Source: CAD feature listing. Evaluate the final solid. Frame: model axes, mm. Face numbers are marked on the shaded views. A direction names the side the tool comes from. Give positions to 0.01 mm unless a question says otherwise; leave off trailing zeros. Order: outer loops, then holes, each group sorted by start corner. A loop starts at its lowest first (then second) coordinate and runs counter-clockwise, first axis right, second up. Notation, with made-up numbers: (77, 19.25) - (116, 19.25) arc R23 cw to (116, 29.25) - close; hole circle Ø8 at (44.5, 71.5). An arc over 180 degrees is marked (long way). Answer as CSV lines item,"result".
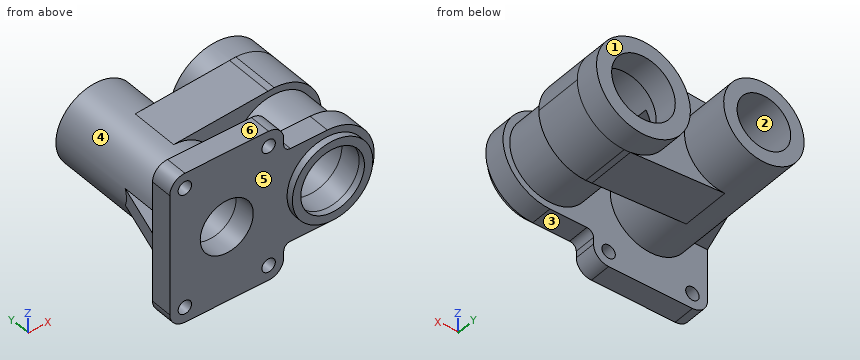
```python
from build123d import *

# Parameters (mm, degrees)
SKETCH3_W                 = 68
SKETCH3_H                 = 90
BOSS_EXTRUDE1_DEPTH       = 13
FILLET2_R                 = 4
FILLET3_R                 = 9
SKETCH5_R                 = 4
CUT_EXTRUDE1_DEPTH        = 100.689518005
SKETCH6_R                 = 24
SKETCH6_R_2               = 16
BOSS_EXTRUDE2_DEPTH       = 41.064418341
SKETCH7_R                 = 24
SKETCH7_R_2               = 19
BOSS_EXTRUDE3_DEPTH       = 17
BOSS_EXTRUDE4_START       = 28
SKETCH7_2_R               = 24
SKETCH7_2_R_2             = 19
BOSS_EXTRUDE4_DEPTH       = 28
BOSS_EXTRUDE11_DEPTH      = 28
BOSS_EXTRUDE11_DEPTH_BACK = 1
SKETCH8_R                 = 24
SKETCH8_R_2               = 16
SKETCH9_W                 = 95
SKETCH9_H                 = 12
CUT_EXTRUDE2_DEPTH        = 12.5
SKETCH10_R                = 24
SKETCH10_R_2              = 16
BOSS_EXTRUDE12_DEPTH      = 29.5
SKETCH12_R                = 28
SKETCH12_R_2              = 19
BOSS_EXTRUDE13_DEPTH      = 14.5
RIB1_REACH                = 141.539
SKETCH13_WALL_W           = 318.21240823
SKETCH13_WALL_H           = 10
SKETCH15_R                = 15.829166104
SKETCH15_R_2              = 19
CUT_EXTRUDE5_DEPTH        = 140.539420953


with BuildPart() as part:
    # Sketch3 → Boss-Extrude1 (new body)
    with BuildSketch(Plane(origin=(0, 0, 0), x_dir=(1, 0, 0), z_dir=(0, 1, 0))):
        Rectangle(SKETCH3_W, SKETCH3_H)
        with BuildLine():
            Line((60, 28), (34, 28))
            Line((34, 28), (34, -28))
            Line((34, -28), (60, -28))
            ThreePointArc((60, -28), (88, 0), (60, 28))
        make_face()
    extrude(amount=BOSS_EXTRUDE1_DEPTH)

    # Fillet2
    fillet2_edges = [part.edges().sort_by_distance(p)[0] for p in [
        (34, 6.5, -28),
        (34, 6.5, 28),
    ]]
    fillet(fillet2_edges, radius=FILLET2_R)

    # Fillet3
    fillet3_edges = [part.edges().sort_by_distance(p)[0] for p in [
        (34, 6.5, 45),
        (-34, 6.5, 45),
        (-34, 6.5, -45),
        (34, 6.5, -45),
    ]]
    fillet(fillet3_edges, radius=FILLET3_R)

    # Sketch5 → Cut-Extrude1 (cut, through all)
    with BuildSketch(Plane(origin=(0, 13, 0), x_dir=(1, 0, 0), z_dir=(0, 1, 0))):
        with Locations(Location((-25, 36, 0), (0, 0, 270))):
            Circle(SKETCH5_R)
        with Locations(Location((25, 36, 0), (0, 0, 270))):
            Circle(SKETCH5_R)
        with Locations(Location((-25, -36, 0), (0, 0, 270))):
            Circle(SKETCH5_R)
        with Locations(Location((25, -36, 0), (0, 0, 270))):
            Circle(SKETCH5_R)
    extrude(amount=-CUT_EXTRUDE1_DEPTH, mode=Mode.SUBTRACT)

    # Sketch6 → Boss-Extrude2 (add)
    with BuildSketch(Plane(origin=(0, 0, 0), x_dir=(1, 0, 0), z_dir=(0, 1, 0))):
        with Locations(Location((0, 0, 0), (0, 0, 270))):
            Circle(SKETCH6_R)
        with Locations(Location((0, 0, 0), (0, 0, 270))):
            Circle(SKETCH6_R_2, mode=Mode.SUBTRACT)
    extrude(amount=BOSS_EXTRUDE2_DEPTH)

    # Sketch7 → Boss-Extrude3 (add)
    with BuildSketch(Plane(origin=(0, 13, 0), x_dir=(1, 0, 0), z_dir=(0, 1, 0))):
        with Locations(Location((60, 0, 0), (0, 0, 270))):
            Circle(SKETCH7_R)
        with Locations(Location((60, 0, 0), (0, 0, 270))):
            Circle(SKETCH7_R_2, mode=Mode.SUBTRACT)
    extrude(amount=-BOSS_EXTRUDE3_DEPTH)

    # Sketch7_2 → Boss-Extrude4 (add)
    with BuildSketch(Plane(origin=(0, 13, 0), x_dir=(1, 0, 0), z_dir=(0, 1, 0)).offset(BOSS_EXTRUDE4_START)):
        with Locations(Location((60, 0, 0), (0, 0, 270))):
            Circle(SKETCH7_2_R)
        with Locations(Location((60, 0, 0), (0, 0, 270))):
            Circle(SKETCH7_2_R_2, mode=Mode.SUBTRACT)
    extrude(amount=-BOSS_EXTRUDE4_DEPTH)

    # Sketch8 → Boss-Extrude11 (add, two sides: drawn at the far end of the back side and taken through both)
    # profile 1 of 3: a face of its own
    with BuildSketch(Plane(origin=(0, 41, 0), x_dir=(1, 0, 0), z_dir=(0, 1, 0)).offset(-BOSS_EXTRUDE11_DEPTH_BACK)):
        with Locations(Location((0, 0, 0), (0, 0, 270))):
            Circle(SKETCH8_R)
        with Locations(Location((0, 0, 0), (0, 0, 270))):
            Circle(SKETCH8_R_2, mode=Mode.SUBTRACT)
    # profile 2 of 3: a face of its own
    with BuildSketch(Plane(origin=(0, 41, 0), x_dir=(1, 0, 0), z_dir=(0, 1, 0)).offset(-BOSS_EXTRUDE11_DEPTH_BACK)):
        with BuildLine():
            Line((60, 28), (56.283185841, 27.752212389))
            ThreePointArc((56.283185841, 27.752212389), (32, 0), (56.283185841, -27.752212389))
            Line((56.283185841, -27.752212389), (60, -28))
            ThreePointArc((60, -28), (79.798989873, -19.798989873), (88, 0))
            ThreePointArc((88, 0), (79.798989873, 19.798989873), (60, 28))
        make_face()
        with Locations(Location((60, 0, 0), (0, 0, 270))):
            Circle(SKETCH8_R, mode=Mode.SUBTRACT)
    # profile 3 of 3: a face of its own
    with BuildSketch(Plane(origin=(0, 41, 0), x_dir=(1, 0, 0), z_dir=(0, 1, 0)).offset(-BOSS_EXTRUDE11_DEPTH_BACK)):
        with BuildLine():
            Line((56.283185841, 27.752212389), (0, 24))
            ThreePointArc((0, 24), (16.970562748, 16.970562748), (24, 0))
            ThreePointArc((24, 0), (16.970562748, -16.970562748), (0, -24))
            Line((0, -24), (56.283185841, -27.752212389))
            ThreePointArc((56.283185841, -27.752212389), (32, 0), (56.283185841, 27.752212389))
        make_face()
    extrude(amount=BOSS_EXTRUDE11_DEPTH + BOSS_EXTRUDE11_DEPTH_BACK)

    # Sketch9 → Cut-Extrude2 (cut, symmetric)
    with BuildSketch(Plane.XY):
        with Locations((31.5, 53.5)):
            Rectangle(SKETCH9_W, SKETCH9_H)
    extrude(amount=CUT_EXTRUDE2_DEPTH, both=True, mode=Mode.SUBTRACT)

    # Sketch10 → Boss-Extrude12 (add)
    with BuildSketch(Plane(origin=(0, 69, 0), x_dir=(1, 0, 0), z_dir=(0, 1, 0))):
        with Locations(Location((0, 0, 0), (0, 0, 270))):
            Circle(SKETCH10_R)
        with Locations(Location((0, 0, 0), (0, 0, 270))):
            Circle(SKETCH10_R_2, mode=Mode.SUBTRACT)
    extrude(amount=BOSS_EXTRUDE12_DEPTH)

    # Sketch12 → Boss-Extrude13 (add)
    with BuildSketch(Plane(origin=(0, 69, 0), x_dir=(1, 0, 0), z_dir=(0, 1, 0))):
        with Locations(Location((60, 0, 0), (0, 0, 270))):
            Circle(SKETCH12_R)
        with Locations(Location((60, 0, 0), (0, 0, 270))):
            Circle(SKETCH12_R_2, mode=Mode.SUBTRACT)
    extrude(amount=BOSS_EXTRUDE13_DEPTH)

    # Sketch13 wall → Rib1 (add, up to next)
    with BuildSketch(Plane(origin=(-28.5, 30.733455303, 0), x_dir=(0.296227943859, 0.955117273049, 0), z_dir=(-0.955117273049, 0.296227943859, 0)), mode=Mode.PRIVATE) as rib1_sk1:
        Rectangle(SKETCH13_WALL_W, SKETCH13_WALL_H)
    rib1_tool1 = extrude(rib1_sk1.sketch, amount=-RIB1_REACH, mode=Mode.PRIVATE) - part.part
    add(rib1_tool1.solids().sort_by_distance((-28.5, 30.733455303, 0))[0])

    # Sketch15 → Cut-Extrude5 (cut, through all)
    with BuildSketch(Plane(origin=(0, 0, 0), x_dir=(1, 0, 0), z_dir=(0, 1, 0))):
        with Locations(Location((0, 0, 0), (0, 0, 270))):
            Circle(SKETCH15_R)
        with Locations(Location((60, 0, 0), (0, 0, 270))):
            Circle(SKETCH15_R_2)
    extrude(amount=CUT_EXTRUDE5_DEPTH, mode=Mode.SUBTRACT)


solid = part.part
```
(1) Contact query for flat-ended pins moving along their axis: pin 1 (6.5 mm diameter, centred on x = -13, z = -8.5, fed in from -Y); pin 2 (14.5 mm diameter, centred on x = 65.5, z = 2.5, fed in from -Y); pin 3 (4 mm diameter, centred on x = 69.5, y = 52.5, fed in from -Z); pin 4 (1.8 mm diameter, centred on x = -12.5, y = 55.5, fed in from -Z). Output: stop coordinate, or through.
Completed:
pin 1,"y = 0"
pin 2,"through"
pin 3,"z = -26.98"
pin 4,"z = -21.01"
(2) Cut plane C-C (y = 56). Return loops of the section in (x, z), then the cut area to 3 significant figures.
Completed:
outline,"(0, -24) - (60, -28) arc R28 ccw to (60, 28) - (0, 24) arc R24 ccw to start; hole (-16, -12.5) - (-9.99, -12.5) arc R16 ccw to (9.99, -12.5) - (39.51, -12.5) arc R24 ccw (long way) to (39.51, 12.5) - (9.99, 12.5) arc R16 ccw to (-9.99, 12.5) - (-16, 12.5) - close"
area,"2,020 mm²"
(3) Mould query, pull axis Y, two halves, no side actions, for the marked faces 4, 5 and 6. Classes: released by +Y, released by -Y, zero draft, split by the parting line, or undercut.
Completed:
face 4,"undercut"
face 5,"released by -Y"
face 6,"zero draft"
(4) Access query for the marked faces 1, 2 and 3. Directions: +Z, -Z, +X, -X, +Y, -Y. A direction counts if a zero-diameter tool reaches every point of the face in a straight line with its end or side. Return the directions, or none.
Completed:
face 1,"+Z, -Z, +X, +Y"
face 2,"+Y"
face 3,"-Z, +X, +Y, -Y"
(5) Cut plane A-A (y = 36). Return loops of the section in (x, z), then the cut area to 3 significant figures.
Completed:
outline,"(-26.87, -5) - (-23.47, -5) arc R24 ccw (long way) to (-23.47, 5) - (-26.87, 5) - close; circle Ø48 at (60, 0); hole circle Ø32 at (0, 0); hole circle Ø38 at (60, 0)"
area,"1,710 mm²"
(6) Cut plane B-B (z = -38). Return loops of the section in (x, y), then the cut area to 3 significant figures.
Completed:
outline,"(-33.77, 0) - (-28.46, 0) - (-28.46, 13) - (-33.77, 13) - close; (-21.54, 0) - (21.54, 0) - (21.54, 13) - (-21.54, 13) - close; (28.46, 0) - (33.77, 0) - (33.77, 13) - (28.46, 13) - close"
area,"698 mm²"
(7) Ray query, line 1 (X direction, y = 4.5, z = -36); line 2 (X direction, y = 47, z = 0); line 3 (Y direction, x = 20, z = 9). Return the intervals inside material, ascending. Write a range as from..to.
Completed:
line 1,"-34..-29, -21..21, 29..34"
line 2,"-24..-16, 16..36, 84..88"
line 3,"0..47.5, 59.5..98.5"
